from build123d import *

# Parameters (mm, degrees)
SKETCH1_W           = 6.35
SKETCH1_H           = 6.35
BOSS_EXTRUDE1_DEPTH = 152.4
SKETCH4_R           = 1.651
CUT_EXTRUDE1_DEPTH  = 12.7
SKETCH5_R           = 1.651
CUT_EXTRUDE2_DEPTH  = 153.565274965


with BuildPart() as part:
    # Sketch1 → Boss-Extrude1 (new, symmetric)
    with BuildSketch(Plane(origin=(0, 0, 0), x_dir=(0, 0, -1), z_dir=(1, 0, 0))):
        Rectangle(SKETCH1_W, SKETCH1_H)
    extrude(amount=BOSS_EXTRUDE1_DEPTH, both=True)

    # Sketch4 → Cut-Extrude1 (cut)
    with BuildSketch(Plane(origin=(152.4, 0, 0), x_dir=(0, 0, -1), z_dir=(1, 0, 0))):
        Circle(SKETCH4_R)
    cut_extrude1 = extrude(amount=-CUT_EXTRUDE1_DEPTH, mode=Mode.SUBTRACT)

    # Sketch5 → Cut-Extrude2 (cut, through all)
    with BuildSketch(Plane.XY.offset(3.175)):
        with Locations((114.3, 0)):
            Circle(SKETCH5_R)
    cut_extrude2 = extrude(amount=-CUT_EXTRUDE2_DEPTH, mode=Mode.SUBTRACT)

    # Mirror1: Cut-Extrude1, Cut-Extrude2 across plane
    add(cut_extrude1.mirror(Plane(origin=(0, 0, 0), x_dir=(0, 0, 1), z_dir=(1, 0, 0))), mode=Mode.SUBTRACT)
    add(cut_extrude2.mirror(Plane(origin=(0, 0, 0), x_dir=(0, 0, 1), z_dir=(1, 0, 0))), mode=Mode.SUBTRACT)


solid = part.part
For this review, take the finished solid that the model builds, in its own axes (mm). Coordinates: 2 decimals unless noted, no trailing zeros. Write each loop counter-clockwise with the first axis right and the second up, starting at its lowest first coordinate (ties: lowest second). Pieces come first, ordered by that corner, then holes. Notation, with made-up numbers: (-36, 48) -> (21, 48) arc R15 ccw to (21, 52) -> close; hole circle Ø9 at (56, -8). An arc over 180 degrees is marked (long way). Write each question's results on one line, items separated by ' | '. Start each with the question number.
1) Insertion check: pin 1 (3 mm diameter, centred on y = 0.5, z = 0.5, fed in from +X); pin 2 (1 mm diameter, centred on y = -0.5, z = -0.5, fed in from +X); pin 3 (2 mm diameter, centred on x = -114.3, y = 0, fed in from -Z); pin 4 (1.7 mm diameter, centred on y = 0, z = -0.5, fed in from -X). Each pin has a flat end and moves straight along its axis. Give the tip position at first contact, or say it passes through.
2) Wall thickness on L1, parallel to Y at x = -114.3, z = -1 (3 decimals); L2, parallel to X at y = 1.5, z = 0; L3, parallel to X at y = -1.25, z = -1: over which ranges is each line inside the solid? List them lowest first. Write a range as [from, to].
3) Consider section A-A (y = 0). Write out the cut boundary in (x, z) (3 decimals).
4) Consider section B-B (z = 0). Write out the cut boundary in (x, y) (3 decimals), plus the area to 3 significant figures.
Geometry says:
1) pin 1: x = 152.4 | pin 2: x = 139.7 | pin 3: through | pin 4: x = -139.7
2) L1: [-3.175, -1.651], [1.651, 3.175] | L2: [-139.7, -114.99], [-113.61, 113.61], [114.99, 139.7] | L3: [-139.7, -115.38], [-113.22, 113.22], [115.38, 139.7]
3) outline: (-152.4, -3.175) -> (-115.951, -3.175) -> (-115.951, 3.175) -> (-152.4, 3.175) -> (-152.4, 1.651) -> (-139.7, 1.651) -> (-139.7, -1.651) -> (-152.4, -1.651) -> close; (-112.649, -3.175) -> (112.649, -3.175) -> (112.649, 3.175) -> (-112.649, 3.175) -> close; (115.951, -3.175) -> (152.4, -3.175) -> (152.4, -1.651) -> (139.7, -1.651) -> (139.7, 1.651) -> (152.4, 1.651) -> (152.4, 3.175) -> (115.951, 3.175) -> close
4) outline: (-152.4, -3.175) -> (152.4, -3.175) -> (152.4, -1.651) -> (139.7, -1.651) -> (139.7, 1.651) -> (152.4, 1.651) -> (152.4, 3.175) -> (-152.4, 3.175) -> (-152.4, 1.651) -> (-139.7, 1.651) -> (-139.7, -1.651) -> (-152.4, -1.651) -> close; hole circle Ø3.302 at (-114.3, 0); hole circle Ø3.302 at (114.3, 0) | area: 1,830 mm^2
